Work out the finished part from the listing and answer in its coordinate system (mm). Face numbers are marked on the shaded views. A direction names the side the tool comes from. Coordinates: 2 decimals unless noted, no trailing zeros. Loops run counter-clockwise (first coordinate to the right, second up) from the corner with the lowest first, then second, coordinate; pieces in that order, holes last. Notation, with made-up numbers: (-31.5, 32.25) - (-4.5, 32.25) arc R19 ccw to (-4.5, 55.25) - close; hole circle Ø3 at (9, 47.5). An arc over 180 degrees is marked (long way). Write each question's results on one line, items separated by ' | '. Start each with the question number.
Item 1: For a pull along Z with two mould halves and no side action, classify the marked faces 1, 2 and 3 as +Z half, -Z half, draft (parallel to the pull), parting line (faces both ways), or undercut.
Item 2: Consider probe 1 along Z at (x, y) = (0, 0.4); probe 2 along Y at (x, z) = (3, -1.75); probe 3 along X at (y, z) = (0.5, -11). Determine where each line is inside the solid, lowest interval first. Write a range as [from, to].
Item 3: Each of these flat-tipped pins is pushed along its axis until it touches: pin 1 Ø1 at (y, z) = (2, -2) entering from +X; pin 2 Ø1.5 at (y, z) = (1, 4.5) entering from +X; pin 3 Ø5.5 at (x, z) = (0, -2) entering from -Y. Where does it stop, or does it pass through?
Item 4: Section B-B, the plane y = 1.3 is taken. Count the separate pieces of the cut face and the enclosed holes in it, plus the area to 3 significant figures.
Item 5: A tool of negligible diameter and unlimited length cuts with its end or side. For the marked faces 4, 5 and 6, from which of +Z, -Z, +X, -X, +Y, -Y can it reach the whole face along a straight path? Write none if from no direction.
Item 6: Section C-C, the plane z = -11.5 is taken. Write down the section's boundary in (x, y).
Item 7: Section A-A, the plane z = 8.75 is taken. Write down the section's boundary in (x, y), plus the area to 3 significant figures.
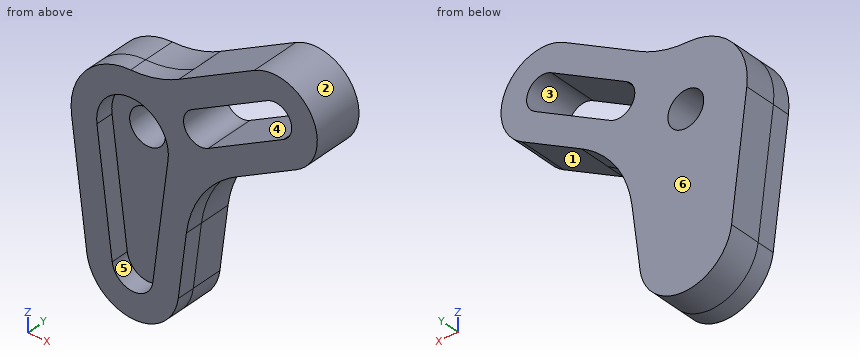
from build123d import *

# Parameters (mm, degrees)
EXTRUDE_THIN1_DEPTH = 1.7
BOSS_EXTRUDE1_DEPTH = 3
EXTRUDE_THIN2_DEPTH = 4.7
FILLET1_R           = 10
SKETCH5_R           = 1.75
CUT_EXTRUDE1_DEPTH  = 25.897593892909114


# Read off the part's stored shape, not the designer's step: Extrude-Thin1
with BuildPart() as part:
    # Extrude-Thin1 outline → Extrude-Thin1 (new body)
    with BuildSketch(Plane(origin=(0, 0, 0), x_dir=(1, 0, 0), z_dir=(0, 1, 0))):
        with BuildLine():
            ThreePointArc((4.464705337, 12.5625), (0, 16.5), (-4.464705337, 12.5625))
            Line((-4.464705337, 12.5625), (-5.95294045, 0.75))
            ThreePointArc((-5.95294045, 0.75), (0, -6), (5.95294045, 0.75))
            Line((5.95294045, 0.75), (4.464705337, 12.5625))
        make_face()
        with BuildLine():
            Line((-3.472548596, 0.4375), (-1.984313483, 12.25))
            ThreePointArc((-1.984313483, 12.25), (0, 14), (1.984313483, 12.25))
            Line((1.984313483, 12.25), (3.472548596, 0.4375))
            ThreePointArc((3.472548596, 0.4375), (0, -3.5), (-3.472548596, 0.4375))
        make_face(mode=Mode.SUBTRACT)
    extrude(amount=EXTRUDE_THIN1_DEPTH)

    # Sketch2 → Boss-Extrude1 (add)
    with BuildSketch(Plane(origin=(0, 1.7, 0), x_dir=(1, 0, 0), z_dir=(0, 1, 0))):
        with BuildLine():
            Line((4.464705337421497, 12.5625), (5.952940449895328, 0.7499999999999997))
            ThreePointArc((5.952940449895328, 0.7499999999999997), (-1.1e-15, -6.000000000000001), (-5.95294044989533, 0.7500000000000003))
            Line((-5.95294044989533, 0.7500000000000003), (-4.464705337421497, 12.562499999999998))
            ThreePointArc((-4.464705337421497, 12.562499999999998), (-7.2e-16, 16.5), (4.464705337421497, 12.5625))
        make_face()
    extrude(amount=BOSS_EXTRUDE1_DEPTH)

    # Sketch4 → Extrude-Thin2 (add, through all)
    with BuildSketch(Plane(origin=(0, 4.7, 0), x_dir=(1, 0, 0), z_dir=(0, 1, 0))):
        with BuildLine():
            Line((8.631793068761734, -0.2492958444837754), (15.993009000929478, -4.499295844483755))
            ThreePointArc((15.99300900092945, -4.499295844483736), (17.49371315644571, -10.099999999999966), (11.893009000929466, -11.600704155516153))
            Line((11.893009000929494, -11.60070415551617), (4.531793068761752, -7.350704155516189))
            ThreePointArc((4.531793068761758, -7.350704155516187), (3.0310889132455334, -1.7499999999999925), (8.631793068761736, -0.24929584448377584))
        make_face()
        with BuildLine():
            Line((7.381793068761741, -2.4143593539448753), (14.743009000929485, -6.664359353944855))
            ThreePointArc((14.743009000929485, -6.664359353944855), (15.328649646984612, -8.849999999999971), (13.143009000929489, -9.43564064605507))
            Line((13.143009000929489, -9.43564064605507), (5.781793068761747, -5.185640646055089))
            ThreePointArc((5.781793068761747, -5.185640646055089), (5.196152422706634, -2.999999999999985), (7.381793068761741, -2.4143593539448753))
        make_face(mode=Mode.SUBTRACT)
    extrude(amount=-EXTRUDE_THIN2_DEPTH)

    # Fillet1
    fillet1_edges = [part.edges().sort_by_distance(p)[0] for p in [
        (5.994462735157251, 3.2, -0.2577140213706832),
        (2.7740444781602016, 3.2, 5.320214021370655),
    ]]
    fillet(fillet1_edges, radius=FILLET1_R)

    # Sketch5 → Cut-Extrude1 (cut, through all)
    with BuildSketch(Plane(origin=(0, 4.7, 0), x_dir=(1, 0, 0), z_dir=(0, 1, 0))):
        with Locations(Location((0, 0, 0), (0, 0, 270))):
            Circle(SKETCH5_R)
    extrude(amount=-CUT_EXTRUDE1_DEPTH, mode=Mode.SUBTRACT)


solid = part.part
Answer key:
1) face 1: -Z half | face 2: parting line | face 3: undercut
2) probe 1: z = [-16.5, -14], [3.5, 6] | probe 2: y = [1.7, 4.7] | probe 3: x = [-4.66, -2.14], [2.14, 4.66]
3) pin 1: stops at x = 7.19 | pin 2: stops at x = 16.94 | pin 3: stops at y = 1.7
4) separate pieces: 1 | enclosed holes: 2 | area: 206 mm^2
5) face 4: +Y, -Y | face 5: -Y | face 6: +Z, -Z, +X, -X, +Y
6) outline: (-4.6, 0) - (-2.08, 0) - (-2.08, 1.7) - (2.08, 1.7) - (2.08, 0) - (4.6, 0) - (4.6, 4.7) - (-4.6, 4.7) - close
7) outline: (6.96, 0) - (11.96, 0) - (11.96, 4.7) - (6.96, 4.7) - close; (15.38, 0) - (17.98, 0) - (17.98, 4.7) - (15.38, 4.7) - close | area: 35.7 mm^2
